Work out the finished part from the listing and answer in its coordinate system (mm). Give positions to 0.01 mm unless a question says otherwise; leave off trailing zeros. Order: outer loops, then holes, each group sorted by start corner. A loop starts at its lowest first (then second) coordinate and runs counter-clockwise, first axis right, second up. Notation, with made-up numbers: (30.5, 89) - (35.5, 89) arc R20 cw to (35.5, 125) - close; hole circle Ø3 at (-4.5, 54.25). An arc over 180 degrees is marked (long way). Write each question's results on one line, items separated by ' | '.
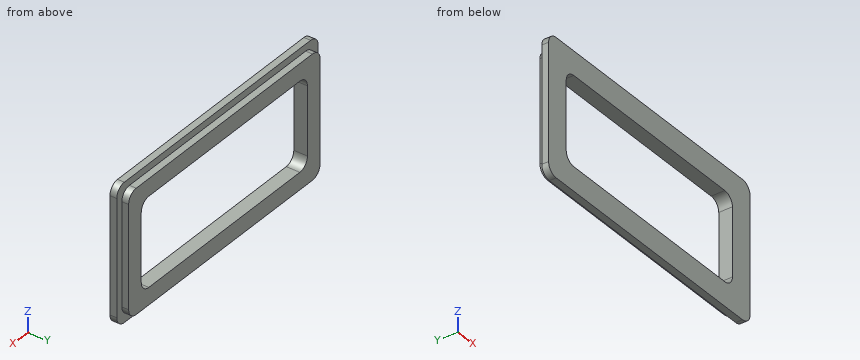
from build123d import *

# Parameters (mm, degrees)
F0_W     = 508
F0_H     = 254
F0_W_2   = 419.1
F0_H_2   = 165.1
F1_DEPTH = 12.7
F2_W     = 482.6
F2_H     = 228.6
F2_W_2   = 419.1
F2_H_2   = 165.1
F3_DEPTH = 12.7
F4_R     = 19.05


with BuildPart() as f1:
    # F0 (on Front) → F1 (new body)
    with BuildSketch(Plane.XZ):
        Rectangle(F0_W, F0_H)
        Rectangle(F0_W_2, F0_H_2, mode=Mode.SUBTRACT)
    extrude(amount=F1_DEPTH)

    # F2 (on Front) → F3 (join)
    with BuildSketch(Plane.XZ):
        Rectangle(F2_W, F2_H)
        Rectangle(F2_W_2, F2_H_2, mode=Mode.SUBTRACT)
    extrude(amount=-F3_DEPTH)

    # F4
    f4_edges = [f1.edges().sort_by_distance(p)[0] for p in [
        (254, -6.35, 127),
        (241.3, 6.35, 114.3),
        (209.55, 0, 82.55),
        (254, -6.35, -127),
        (241.3, 6.35, -114.3),
        (209.55, 0, -82.55),
        (-209.55, 0, -82.55),
        (-241.3, 6.35, -114.3),
        (-254, -6.35, -127),
        (-254, -6.35, 127),
        (-241.3, 6.35, 114.3),
        (-209.55, 0, 82.55),
    ]]
    fillet(f4_edges, radius=F4_R)


solid = f1.part
1. Straight lines are drawn through the part: line 1 (Z direction, x = 34, y = 0.75); line 2 (X direction, y = -10.5, z = 20.5); line 3 (Z direction, x = 186, y = -1.75). For each, find the intervals that lie inside material, in ascending order. Write a range as [from, to].
Answer list:
line 1: [-114.3, -82.55], [82.55, 114.3] | line 2: [-254, -209.55], [209.55, 254] | line 3: [-127, -82.55], [82.55, 127]
2. A cutting plane is placed at A-A, the plane z = -41.5. Write down the section's boundary in (x, y).
Answer list:
outline: (-254, -12.7) - (-209.55, -12.7) - (-209.55, 12.7) - (-241.3, 12.7) - (-241.3, 0) - (-254, 0) - close; (209.55, -12.7) - (254, -12.7) - (254, 0) - (241.3, 0) - (241.3, 12.7) - (209.55, 12.7) - close
3. A cutting plane is placed at B-B, the plane x = -172. Write down the section's boundary in (y, z), then the cut area to 3 significant figures.
Answer list:
outline: (-12.7, -127) - (0, -127) - (0, -114.3) - (12.7, -114.3) - (12.7, -82.55) - (-12.7, -82.55) - close; (-12.7, 82.55) - (12.7, 82.55) - (12.7, 114.3) - (0, 114.3) - (0, 127) - (-12.7, 127) - close | area: 1,940 mm^2
4. Given P1, Ø12.5, axis at y = 5, z = -15, coming from the -X side; P2, Ø1, axis at y = 3.5, z = -41.5, coming from the +X side; P3, Ø2, axis at x = -173.5, y = 2, coming from the -Z side, each flat-ended and moving along its own axis, determine where each tip first touches the part or whether it passes through.
Answer list:
P1: x = -254 | P2: x = 241.3 | P3: z = -114.3
